Verification items for the finished model (mm, model axes). Give positions to 0.01 mm unless a question says otherwise; leave off trailing zeros. Loops run counter-clockwise (first coordinate to the right, second up) from the corner with the lowest first, then second, coordinate; pieces in that order, holes last. Notation, with made-up numbers: (18, 62) - (26, 62) arc R23 cw to (26, 97) - close; hole circle Ø7 at (13, 41.25). An arc over 180 degrees is marked (long way). Answer in a Markdown table with one row per item.
```python
from build123d import *

# Parameters (mm, degrees)
F0_W     = 105.567920953
F0_H     = 76.1951208115
F1_DEPTH = 76.2
F2_T     = -2.54
F3_W     = 105.567920953
F3_H     = 73.66
F3_W_2   = 85.8121328056
F3_H_2   = 57.7212069184
F4_DEPTH = 1.905


with BuildPart() as f1:
    # F0 (on Top) → F1 (new body)
    with BuildSketch(Plane.XY):
        with Locations((7.5357314199, -38.0975604057)):
            Rectangle(F0_W, F0_H)
    extrude(amount=F1_DEPTH)

    # F2
    f2_openings = [f1.faces().sort_by_distance(p)[0] for p in [
        (7.535731, -38.09756, 76.2),
        (7.535731, -76.195121, 38.1),
        (-45.248229, -38.09756, 38.1),
        (60.319692, -38.09756, 38.1),
    ]]
    offset(amount=F2_T, openings=f2_openings)

    # F3 (on face) → F4 (join)
    with BuildSketch(Plane.XZ.offset(2.54)):
        with Locations((7.5357314199, 39.37)):
            Rectangle(F3_W, F3_H)
        with Locations((7.8303422779, 39.7484777495)):
            Rectangle(F3_W_2, F3_H_2, mode=Mode.SUBTRACT)
    extrude(amount=F4_DEPTH)


solid = f1.part
```
Q1. Draft check along Z on faces 1 (the face through (7, -4.445, 73)), 2 (the face through (7, -2.54, 39)), 3 (the face through (7, -40, 2.54)). Enter one of: +Z half, -Z half, draft (parallel to the pull), parting line (faces both ways), or undercut.
Completed:
| item | result |
|---|---|
| face 1 | draft |
| face 2 | undercut |
| face 3 | +Z half |
Q2. Go/stop test with flat-tipped pins: P1, Ø22, axis at x = -15, z = 39.5, coming from the -Y side; P2, Ø4, axis at x = 14.5, y = -68, coming from the +Z side. Record where each tip stops, or that it passes through.
Completed:
| item | result |
|---|---|
| P1 | y = -2.54 |
| P2 | z = 2.54 |
Q3. Thickness scan on line 1 (Z direction, x = 12, y = -35); line 2 (Y direction, x = -16, z = 67.5); line 3 (Y direction, x = 5, z = 5.5) (3 decimals). Record the ranges inside material, lowest first.
Completed:
| item | result |
|---|---|
| line 1 | 0 to 2.54 |
| line 2 | -2.54 to 0 |
| line 3 | -4.445 to 0 |
Q4. Sectioned sample at A-A (z = 18.5). Record the cut outline in (x, y) (3 decimals).
Completed:
| item | result |
|---|---|
| outline | (-45.248, -4.445) - (-35.076, -4.445) - (-35.076, -2.54) - (50.736, -2.54) - (50.736, -4.445) - (60.32, -4.445) - (60.32, 0) - (-45.248, 0) - close |
Q5. Sectioned sample at C-C (y = -14). Record the cut outline in (x, z), and give its area (3 significant figures).
Completed:
| item | result |
|---|---|
| outline | (-45.25, 0) - (60.32, 0) - (60.32, 2.54) - (-45.25, 2.54) - close |
| area | 268 mm^2 |
Q6. Sectioned sample at B-B (x = 52). Record the cut outline in (y, z) (3 decimals), and give its area (3 significant figures).
Completed:
| item | result |
|---|---|
| outline | (-76.195, 0) - (0, 0) - (0, 76.2) - (-4.445, 76.2) - (-4.445, 2.54) - (-76.195, 2.54) - close |
| area | 521 mm^2 |
Q7. Sectioned sample at D-D (z = 71). Record the cut outline in (x, y) (3 decimals).
Completed:
| item | result |
|---|---|
| outline | (-45.248, -4.445) - (60.32, -4.445) - (60.32, 0) - (-45.248, 0) - close |
